Geometry check sheet. Reference: drawing and pictorial views, mm from the part's lowest x, y, z. A direction names the side the tool comes from. Round coordinates to 2 decimals unless told otherwise and drop trailing zeros. Write each loop counter-clockwise with the first axis right and the second up, starting at its lowest first coordinate (ties: lowest second). Pieces come first, ordered by that corner, then holes. Notation, with made-up numbers: (-1.5, 49.5) -> (56.5, 49.5) arc R10 ccw to (56.5, 58.5) -> close; hole circle Ø10 at (14, -5.5). An arc over 180 degrees is marked (long way). Answer as a JSON object with one key per item and string values. Group by question number.
(1) Draft check along X on the marked faces 4, 5 and 6. Enter one of: released by +X, released by -X, zero draft, split by the parting line, or undercut.
(2) Sectioned sample at C-C on z = 23.5. Record the cut outline in (x, y), and give its area (3 significant figures).
(3) Sectioned sample at B-B on x = 7.5. Record the cut outline in (y, z), and give its area (3 significant figures).
(4) Set-up check for the marked faces 1, 2 and 3: record each of +Z, -Z, +X, -X, +Y, -Y from which the full face is reachable in a straight line by a thin tool's end or side.
(5) Sectioned sample at D-D on y = 1. Record the cut outline in (x, z), and give its area (3 significant figures).
(6) Scan lines: L1, parallel to Y at x = 63.5, z = 35.7; L2, parallel to Z at x = 6.5, y = 3; L3, parallel to Z at x = 36, y = 8.25. Record each from-to range of solid material in increasing order. Write a range as from..to.
(7) Gauge pin test, flat ends, axial feed: pin 1 Ø8 at (y, z) = (2.5, 12) entering from +X; pin 2 Ø1.5 at (y, z) = (1.5, 20) entering from +X; pin 3 Ø8.5 at (x, y) = (7.5, 7.25) entering from -Z. Record the tip position at first contact, or that the pin passes through.
(8) Sectioned sample at A-A on y = 7.25. Record the cut outline in (x, z).
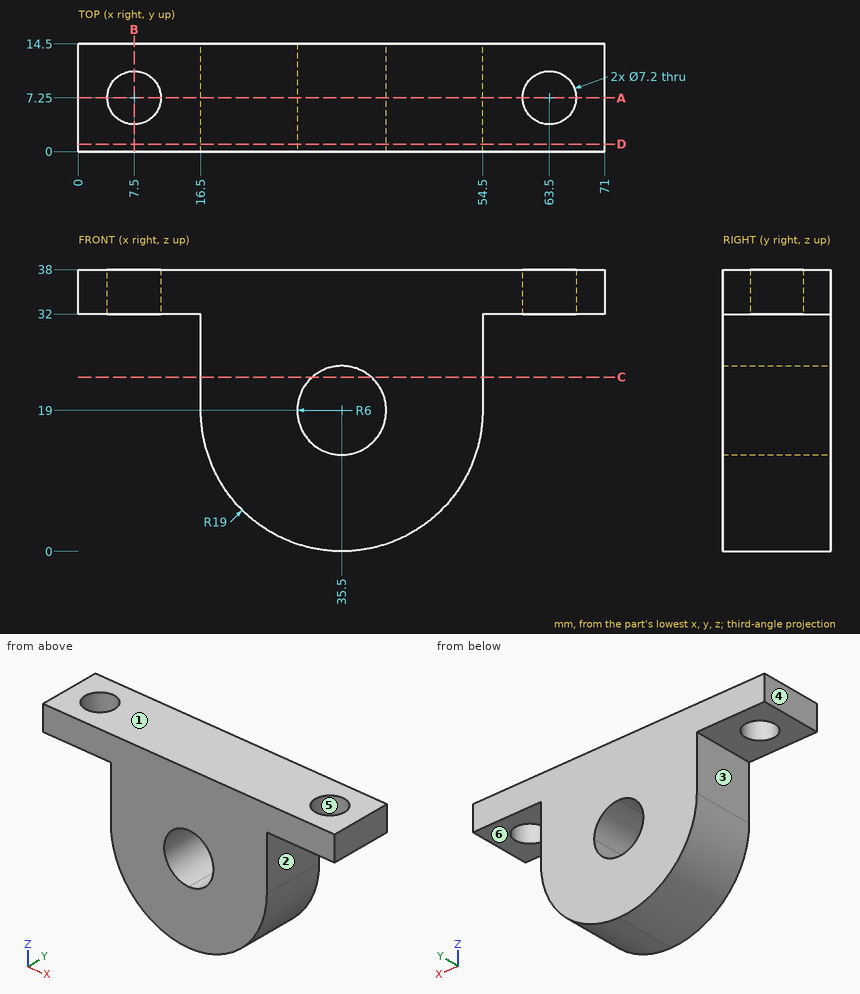
Computed values:
{
 "1": {"face 4": "released by -X", "face 5": "undercut", "face 6": "zero draft"},
 "2": {"outline": "(16.5, 0) -> (31.53, 0) -> (31.53, 14.5) -> (16.5, 14.5) -> close; (39.47, 0) -> (54.5, 0) -> (54.5, 14.5) -> (39.47, 14.5) -> close", "area": "436 mm2"},
 "3": {"outline": "(0, 32) -> (3.65, 32) -> (3.65, 38) -> (0, 38) -> close; (10.85, 32) -> (14.5, 32) -> (14.5, 38) -> (10.85, 38) -> close", "area": "43.8 mm2"},
 "4": {"face 1": "+Z, +X, -X, +Y, -Y", "face 2": "-Z, +X, +Y, -Y", "face 3": "-Z, -X, +Y, -Y"},
 "5": {"outline": "(0, 32) -> (16.5, 32) -> (16.5, 19) arc R19 ccw to (54.5, 19) -> (54.5, 32) -> (71, 32) -> (71, 38) -> (0, 38) -> close; hole circle Ø12 at (35.5, 19)", "area": "1,370 mm2"},
 "6": {"L1": "0..3.65, 10.85..14.5", "L2": "32..38", "L3": "0.01..13.02, 24.98..38"},
 "7": {"pin 1": "x = 54.26", "pin 2": "x = 54.5", "pin 3": "z = 32"},
 "8": {"outline": "(0, 32) -> (3.9, 32) -> (3.9, 38) -> (0, 38) -> close; (11.1, 32) -> (16.5, 32) -> (16.5, 19) arc R19 ccw to (54.5, 19) -> (54.5, 32) -> (59.9, 32) -> (59.9, 38) -> (11.1, 38) -> close; (67.1, 32) -> (71, 32) -> (71, 38) -> (67.1, 38) -> close; hole circle Ø12 at (35.5, 19)"}
}
